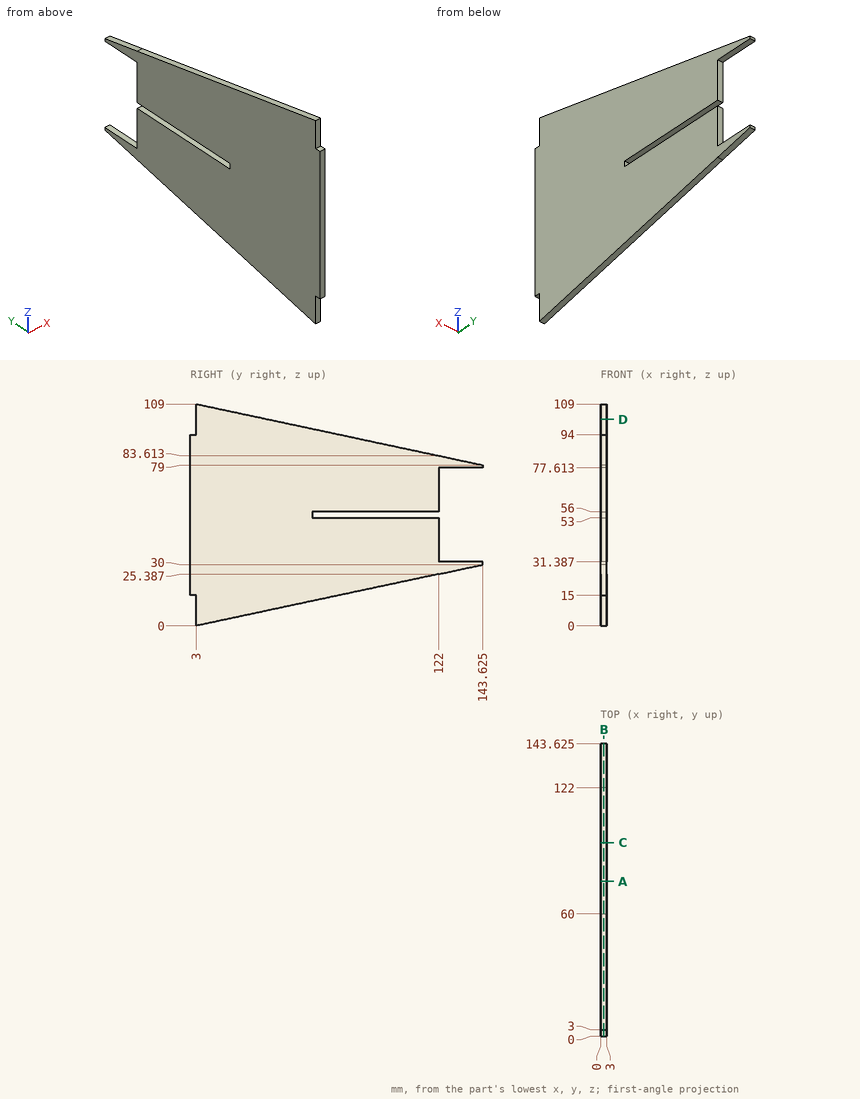
Source: three-view drawing plus pictorial views. Frame: mm from the lowest corner of the part. Round coordinates to 2 decimals unless told otherwise and drop trailing zeros. Write each loop counter-clockwise with the first axis right and the second up, starting at its lowest first coordinate (ties: lowest second). Pieces come first, ordered by that corner, then holes. Notation, with made-up numbers: (70.5, -18) -> (100.5, -18) arc R31 cw to (100.5, 8) -> close; hole circle Ø8 at (83.5, 65). An arc over 180 degrees is marked (long way). Return JSON: item names as keys, results as strings.
Q1. Section D-D on z = 101.5. Return the cut outline in (x, y).
From the geometry:
{"outline": "(0, 3) -> (3, 3) -> (3, 38.16) -> (0, 38.16) -> close"}
Q2. First-contact query: pin 1 Ø0.9 at (x, z) = (1.5, 7.5) entering from -Y; pin 2 Ø1.5 at (x, y) = (2, 87.5) entering from -Z; pin 3 Ø1.5 at (x, z) = (1, 46.5) entering from +Y. Flat tips, straight axial feed; report the tip coordinate or a pass-through.
From the geometry:
{"pin 1": "y = 3", "pin 2": "z = 17.87", "pin 3": "y = 122"}
Q3. Section A-A on y = 76. Return the cut outline in (x, z).
From the geometry:
{"outline": "(0, 15.57) -> (3, 15.57) -> (3, 53) -> (0, 53) -> close; (0, 56) -> (3, 56) -> (3, 93.43) -> (0, 93.43) -> close"}
Q4. Section B-B on x = 1.65. Return the cut outline in (y, z) (1 decimal), and give its area (3 significant figures).
From the geometry:
{"outline": "(0, 15) -> (3, 15) -> (3, 0) -> (143.6, 30) -> (143.6, 31.4) -> (122, 31.4) -> (122, 53) -> (60, 53) -> (60, 56) -> (122, 56) -> (122, 77.6) -> (143.6, 77.6) -> (143.6, 79) -> (3, 109) -> (3, 94) -> (0, 94) -> close", "area": "10,200 mm2"}
Q5. Ray query, line 1 (Z direction, x = 1.35, y = 109); line 2 (Z direction, x = 0.8, y = 97); line 3 (Y direction, x = 1, z = 53.5). Return the intervals inside material, ascending.
From the geometry:
{"line 1": "22.61 to 53, 56 to 86.39", "line 2": "20.05 to 53, 56 to 88.95", "line 3": "0 to 60"}
Q6. Section C-C on y = 95. Return the cut outline in (x, z), and give its area (3 significant figures).
From the geometry:
{"outline": "(0, 19.63) -> (3, 19.63) -> (3, 53) -> (0, 53) -> close; (0, 56) -> (3, 56) -> (3, 89.37) -> (0, 89.37) -> close", "area": "200 mm2"}
